from build123d import *

# Parameters (mm, degrees)
SKETCH1_R           = 3
BOSS_EXTRUDE1_DEPTH = 10
SKETCH2_R           = 5
BOSS_EXTRUDE2_DEPTH = 5
FILLET1_R           = 1


# Read off the part's stored shape, not the designer's step: M5 Machine Threads Stud1
with BuildPart() as part:
    # Sketch1 → Boss-Extrude1 (new body)
    with BuildSketch(Plane(origin=(0, 0, 0), x_dir=(1, 0, 0), z_dir=(0, 1, 0))):
        with Locations(Location((0, 0, 0), (0, 0, 270))):
            Circle(SKETCH1_R)
    extrude(amount=BOSS_EXTRUDE1_DEPTH)

    # Sketch2 → Boss-Extrude2 (add)
    with BuildSketch(Plane(origin=(0, 10, 0), x_dir=(1, 0, 0), z_dir=(0, 1, 0))):
        with Locations(Location((0, 0, 0), (0, 0, 270))):
            Circle(SKETCH2_R)
    extrude(amount=BOSS_EXTRUDE2_DEPTH)

    # Fillet1
    fillet1_edges = [part.edges().sort_by_distance(p)[0] for p in [
        (0, 15, -5),
    ]]
    fillet(fillet1_edges, radius=FILLET1_R)

    # M5 Machine Threads Stud1 outline → M5 Machine Threads Stud1 (revolve, cut)
    with BuildSketch(Plane.XY):
        Polygon((3, 10), (2.5, 10), (2.5, 0.445), (2.055, 0), (3, 0), align=None)
    revolve(axis=Axis((0, 0, 0), (0, 1, 0)), mode=Mode.SUBTRACT)


solid = part.part
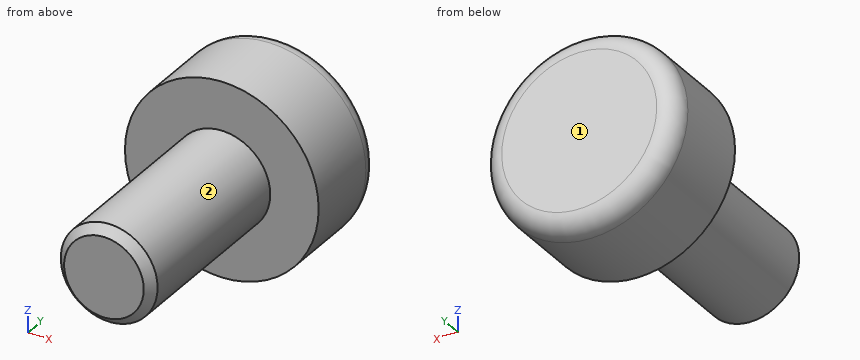
CAD build for the part. Positions are in the model's coordinates, mm. Face numbers are marked on the shaded views. A direction names the side the tool comes from. Coordinates: 2 decimals unless noted, no trailing zeros. Loops run counter-clockwise (first coordinate to the right, second up) from the corner with the lowest first, then second, coordinate; pieces in that order, holes last. Notation, with made-up numbers: (14.25, -25.75) - (45.25, -25.75) arc R13 ccw to (45.25, -15.75) - close; hole circle Ø3 at (39, 12.25). An arc over 180 degrees is marked (long way). Write item = value, one per line. Start each with the question number.
Q1. Cut at A-A, the plane z = 0. List the corners of the cut face in (x, y) (3 decimals).
Q2. Drill centre lines: L1, parallel to Y at x = 1.5, z = 2.5; L2, parallel to X at y = 1.25, z = 0; L3, parallel to X at y = 8.5, z = 1.5. Where is each one in solid material? Low to high.
Q3. Flat gauge pins, fed straight in: pin 1 Ø5 at (x, z) = (3.5, -0.5) entering from -Y; pin 2 Ø5 at (y, z) = (9.5, 3) entering from +X. Where does each tip first touch, or does it go through?
Q4. Which spindle directions (+Z, -Z, +X, -X, +Y, -Y) get a long thin tool onto all of the face, cutting with end or side? Do the marked faces 1 and 2. Say none if no direction does.
Q5. Cut at C-C, the plane y = 5. List the corners of the cut face in (x, z), then the cut area to 3 significant figures.
Q6. Cut at B-B, the plane x = 0. List the corners of the cut face in (y, z) (3 decimals).
Computed:
q1.outline = (-5, 10) - (-2.5, 10) - (-2.5, 0.445) - (-2.055, 0) - (2.055, 0) - (2.5, 0.445) - (2.5, 10) - (5, 10) - (5, 14) arc R1 ccw to (4, 15) - (-4, 15) arc R1 ccw to (-5, 14) - close
q2.L1 = 10 to 15
q2.L2 = -2.5 to 2.5
q2.L3 = -2 to 2
q3.pin_1 = 0
q3.pin_2 = 4.97
q4.face_1 = +Z, -Z, +X, -X, +Y
q4.face_2 = -Y
q5.outline = circle Ø5 at (0, 0)
q5.area = 19.6 mm²
q6.outline = (0, -2.055) - (0.445, -2.5) - (10, -2.5) - (10, -5) - (14, -5) arc R1 ccw to (15, -4) - (15, 4) arc R1 ccw to (14, 5) - (10, 5) - (10, 2.5) - (0.445, 2.5) - (0, 2.055) - close
